Source: CAD feature listing. Evaluate the final solid. Frame: model axes, mm. Face numbers are marked on the shaded views. A direction names the side the tool comes from. Give positions to 0.01 mm unless a question says otherwise; leave off trailing zeros. Loops run counter-clockwise (first coordinate to the right, second up) from the corner with the lowest first, then second, coordinate; pieces in that order, holes last. Notation, with made-up numbers: (59.25, -35.5) -> (88.25, -35.5) arc R15 ccw to (88.25, -27.5) -> close; hole circle Ø11 at (75, -8). An arc over 180 degrees is marked (long way). Answer as a JSON object with one key per item and string values. Group by question number.
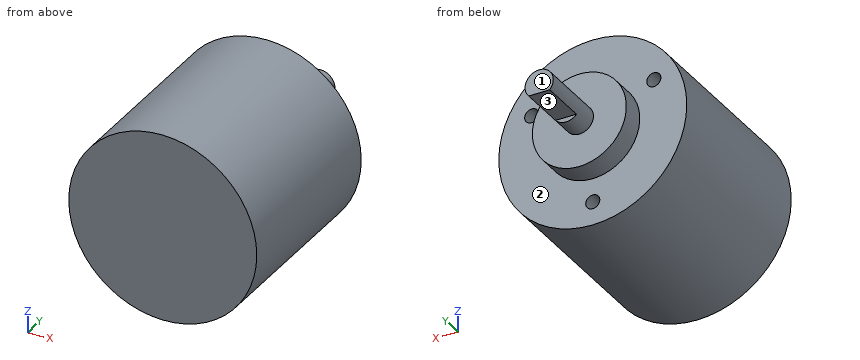
Autodesk Inventor part; units mm, degrees
ref_plane "YZ Plane" through (0, 0, 0) normal (1, 0, 0) x (0, 1, 0)
ref_plane "XZ Plane" through (0, 0, 0) normal (0, 1, 0) x (-1, 0, 0)
ref_plane "XY Plane" through (0, 0, 0) normal (0, 0, 1) x (1, 0, 0)
sketch "Esquisse1" plane through (0, 0, 0) normal (0, 1, 0) x (-1, 0, 0)
  circle A0 centre (0, 0) radius 20
  dimension "d0" = 40
extrude "Extrusion1" add sketch "Esquisse1" along normal blind 39
sketch "Esquisse2" plane through (0, 39, 0) normal (0, 1, 0) x (1, 0, 0)
  circle A0 centre (0, 0) radius 20
  circle A1 centre (0, 0) radius 10
  dimension "d3" = 20
extrude "Extrusion2" add sketch "Esquisse2" along normal blind 5 contours A1
sketch "Esquisse3" plane through (0, 44, 0) normal (0, 1, 0) x (1, 0, 0)
  circle A0 centre (0, 0) radius 10
  circle A1 centre (0, 0) radius 3
  dimension "d6" = 6
extrude "Extrusion3" add sketch "Esquisse3" along normal blind 15 contours A1
sketch "Esquisse4" plane through (0, 59, 0) normal (0, 1, 0) x (1, 0, 0)
  circle A0 centre (0, 0) radius 3 construction
  line L0 (-2.2361, 2) -> (2.2361, 2)
  line L1 (2.2361, 2) -> (2.2361, -2) construction
  line L2 (2.2361, -2) -> (-2.2361, -2) construction
  line L3 (-2.2361, -2) -> (-2.2361, 2) construction
  arc A1 (-2.2361, 2) -> (2.2361, 2) centre (0, 0) ccw
  arc A2 (2.2361, 2) -> (-2.2361, 2) centre (0, 0) ccw
  dimension "d9" = 4
extrude "Extrusion4" cut sketch "Esquisse4" against normal blind 10 contours A2 L0
sketch "Esquisse5" plane through (0, 39, 0) normal (0, 1, 0) x (1, 0, 0)
  circle A0 centre (0, 0) radius 10
  circle A1 centre (0, 0) radius 20
  circle A2 centre (0, 0) radius 15 construction
  circle A3 centre (0, 15) radius 1.5
  circle A4 centre (-12.9904, -7.5) radius 1.5
  circle A5 centre (12.9904, -7.5) radius 1.5
  dimension "d12" = 30
  dimension "d13" = 3
  dimension "d16" = 360
extrude "Extrusion5" cut sketch "Esquisse5" against normal blind 5 contours A3 | A4 | A5
properties part number "encoder_E6B2"
(1) Material intervals for line 1 (Z direction, x = 0, y = 35.9); line 2 (Y direction, x = 14, z = 10.5); line 3 (X direction, y = 37, z = 7) (3 decimals), sorted ascending. Write a range as from..to.
(2) Section query B-B on x = 0. Return the cut outline in (y, z).
(3) Section query D-D on y = 51. Return the cut outline in (x, z), plus the area to 3 significant figures.
(4) Section query C-C on z = 7.5. Return the cut outline in (x, y).
(5) Section query A-A on y = 38. Return the cut outline in (x, z).
(6) First-contact query: pin 1 (6 mm diameter, centred on x = -0.5, y = 6.5, fed in from -Z); pin 2 (1.5 mm diameter, centred on x = 13, z = 7.5, fed in from +Y); pin 3 (3.5 mm diameter, centred on x = -0.5, z = -15.5, fed in from +Y). Flat tips, straight axial feed; report the tip coordinate or a pass-through.
(7) Access query for the marked faces 1, 2 and 3. Directions: +Z, -Z, +X, -X, +Y, -Y. A direction counts if a zero-diameter tool reaches every point of the face in a straight line with its end or side. Return the directions, or none.
Result:
{
 "1": {"line 1": "-20..-16.5, -13.5..20", "line 2": "0..39", "line 3": "-18.735..-14.405, -11.576..11.576, 14.405..18.735"},
 "2": {"outline": "(0, -20) -> (39, -20) -> (39, -16.5) -> (34, -16.5) -> (34, -13.5) -> (39, -13.5) -> (39, -10) -> (44, -10) -> (44, -3) -> (49, -3) -> (49, -2) -> (59, -2) -> (59, 3) -> (44, 3) -> (44, 10) -> (39, 10) -> (39, 20) -> (0, 20) -> close"},
 "3": {"outline": "(-2.24, -2) -> (2.24, -2) arc R3 ccw (long way) to start", "area": "25.2 mm²"},
 "4": {"outline": "(-18.54, 0) -> (18.54, 0) -> (18.54, 39) -> (14.49, 39) -> (14.49, 34) -> (11.49, 34) -> (11.49, 39) -> (6.61, 39) -> (6.61, 44) -> (-6.61, 44) -> (-6.61, 39) -> (-11.49, 39) -> (-11.49, 34) -> (-14.49, 34) -> (-14.49, 39) -> (-18.54, 39) -> close"},
 "5": {"outline": "circle Ø40 at (0, 0); hole circle Ø3 at (-12.99, 7.5); hole circle Ø3 at (0, -15); hole circle Ø3 at (12.99, 7.5)"},
 "6": {"pin 1": "z = -20", "pin 2": "y = 34", "pin 3": "y = 39"},
 "7": {"face 1": "+Z, -Z, +X, -X, +Y", "face 2": "+Y", "face 3": "-Z, +X, -X, +Y"}
}
